Verification items for the finished model (mm, model axes). Face numbers are marked on the shaded views. A direction names the side the tool comes from. Coordinates: 2 decimals unless noted, no trailing zeros. Order: outer loops, then holes, each group sorted by start corner. A loop starts at its lowest first (then second) coordinate and runs counter-clockwise, first axis right, second up. Notation, with made-up numbers: M -4.75,50.5 L 4.25,50.5 A24 ccw 4.25,61.5 Z; hole C 54,45 d9. An arc over 180 degrees is marked long. Return JSON: item names as keys, results as strings. Group by question number.
1. Material ranges on line 1 along Y through (x, z) = (2, 40); line 2 along Z through (x, y) = (-2, 44.75); line 3 along X through (y, z) = (43.5, 56.5), recorded low to high.
2. Set-up check for the marked faces 1, 2, 3, 4 and 5: record each of +Z, -Z, +X, -X, +Y, -Y from which the full face is reachable in a straight line by a thin tool's end or side.
3. Section check D-D, the plane y = 25.75. Record the cut outline in (x, z), plus the area to 3 significant figures.
4. Section check A-A, the plane x = 13.5. Record the cut outline in (y, z).
5. Gauge pin test, flat ends, axial feed: pin 1 (10 mm diameter, centred on x = 41.5, y = 33.5, fed in from -Z); pin 2 (12 mm diameter, centred on y = 34, z = 67.5, fed in from +X); pin 3 (4.5 mm diameter, centred on y = 42, z = 56.5, fed in from -X); pin 4 (3 mm diameter, centred on x = -26, y = 39.5, fed in from +Z). Record the tip position at first contact, or that the pin passes through.
6. Section check B-B, the plane z = 76. Record the cut outline in (x, y).
Solid Edge part; units mm, degrees
sketch "Sketch1" plane through (0, 0, 0) normal (0, 0, 1) x (1, 0, 0)
  line L0 (-47.7385, 17.1455) -> (52.2615, 17.1455)
  line L1 (52.2615, 17.1455) -> (52.2615, 47.1455)
  line L2 (52.2615, 47.1455) -> (-47.7385, 47.1455)
  line L3 (-47.7385, 47.1455) -> (-47.7385, 17.1455)
extrude "Protrusion1" add sketch "Sketch1" along normal blind 30
sketch "Sketch2" plane through (2.2615, 32.1455, 30) normal (0, 0, 1) x (1, 0, 0)
  line L0 (-25, 15) -> (-25, 0)
  line L1 (-25, 0) -> (25, 0)
  line L2 (25, 0) -> (25, 15)
extrude "ExtrudedProtrusion_2" add sketch "Sketch2" along normal blind 75 material side at (-22.6885, 39.6455, 30)
sketch "Sketch3" plane through (2.2615, 32.1455, 67.5) normal (0, -1, 0) x (1, 0, 0)
  circle A0 centre (0, 19.4008) radius 15
extrude "ExtrudedCutout_1" cut sketch "Sketch3" against normal blind 235.9041
fillet "Round_1" radius 25 2 edges at (27.2615, 39.6455, 105) (-22.7385, 39.6455, 105)
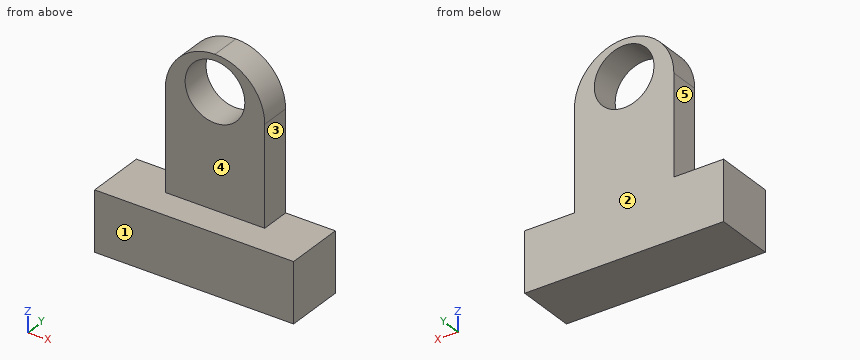
Answers follow:
{
 "1": {"line 1": "32.15 to 47.15", "line 2": "0 to 72.52, 101.28 to 104.63", "line 3": "-22.74 to 27.26"},
 "2": {"face 1": "+Z, -Z, +X, -X, -Y", "face 2": "+Z, -Z, +X, -X, +Y", "face 3": "+Z, +X, +Y, -Y", "face 4": "+Z, +X, -X, -Y", "face 5": "+Z, -X, +Y, -Y"},
 "3": {"outline": "M -47.74,0 L 52.26,0 L 52.26,30 L -47.74,30 Z", "area": "3,000 mm^2"},
 "4": {"outline": "M 17.15,0 L 47.15,0 L 47.15,76.97 L 32.15,76.97 L 32.15,30 L 17.15,30 Z; M 32.15,96.84 L 47.15,96.84 L 47.15,102.33 L 32.15,102.33 Z"},
 "5": {"pin 1": "z = 0", "pin 2": "x = 27.26", "pin 3": "x = -22.74", "pin 4": "z = 30"},
 "6": {"outline": "M -22.74,32.15 L -8.04,32.15 L -8.04,47.15 L -22.74,47.15 Z; M 12.57,32.15 L 27.26,32.15 L 27.26,47.15 L 12.57,47.15 Z"}
}
